```python
from build123d import *

# Parameters (mm, degrees)
SKETCH3_W           = 145
SKETCH3_H           = 90
SKETCH3_W_2         = 141.777777778
SKETCH3_H_2         = 88
BOSS_EXTRUDE1_DEPTH = 110
SKETCH4_W           = 145
SKETCH4_H           = 90
BOSS_EXTRUDE2_DEPTH = 1
SKETCH5_W           = 12
SKETCH5_H           = 12
BOSS_EXTRUDE3_DEPTH = 110
SKETCH6_R           = 2
CUT_EXTRUDE1_DEPTH  = 12
SKETCH7_R           = 10
CUT_EXTRUDE2_DEPTH  = 12


with BuildPart() as part:
    # Sketch3 → Boss-Extrude1 (new body)
    with BuildSketch(Plane(origin=(0, 0, 0), x_dir=(1, 0, 0), z_dir=(0, 1, 0))):
        Rectangle(SKETCH3_W, SKETCH3_H)
        Rectangle(SKETCH3_W_2, SKETCH3_H_2, mode=Mode.SUBTRACT)
    extrude(amount=BOSS_EXTRUDE1_DEPTH)

    # Sketch4 → Boss-Extrude2 (add)
    with BuildSketch(Plane.XZ):
        Rectangle(SKETCH4_W, SKETCH4_H)
    extrude(amount=BOSS_EXTRUDE2_DEPTH)

    # Sketch5 → Boss-Extrude3 (add)
    with BuildSketch(Plane(origin=(0, 0, 0), x_dir=(1, 0, 0), z_dir=(0, 1, 0))):
        with Locations((-64.888888889, 38)):
            Rectangle(SKETCH5_W, SKETCH5_H)
        with Locations((64.888888889, 38)):
            Rectangle(SKETCH5_W, SKETCH5_H)
        with Locations((64.888888889, -38)):
            Rectangle(SKETCH5_W, SKETCH5_H)
        with Locations((-64.888888889, -38)):
            Rectangle(SKETCH5_W, SKETCH5_H)
    extrude(amount=BOSS_EXTRUDE3_DEPTH)

    # Sketch6 → Cut-Extrude1 (cut)
    with BuildSketch(Plane(origin=(0, 110, 0), x_dir=(1, 0, 0), z_dir=(0, 1, 0))):
        with Locations((-67.5, 40)):
            Circle(SKETCH6_R)
        with Locations((-67.5, -40)):
            Circle(SKETCH6_R)
        with Locations((67.5, -40)):
            Circle(SKETCH6_R)
        with Locations((67.5, 40)):
            Circle(SKETCH6_R)
    extrude(amount=-CUT_EXTRUDE1_DEPTH, mode=Mode.SUBTRACT)

    # Sketch7 → Cut-Extrude2 (cut)
    with BuildSketch(Plane(origin=(0, 0, 0), x_dir=(1, 0, 0), z_dir=(0, 1, 0))):
        Circle(SKETCH7_R)
    extrude(amount=-CUT_EXTRUDE2_DEPTH, mode=Mode.SUBTRACT)


solid = part.part
```
Check sheet for the modelled part. Datum: model origin and axes. Units: mm. A direction names the side the tool comes from. Give positions to 0.01 mm unless a question says otherwise; leave off trailing zeros. Order: outer loops, then holes, each group sorted by start corner. A loop starts at its lowest first (then second) coordinate and runs counter-clockwise, first axis right, second up. Notation, with made-up numbers: M -38,10 L -24,10 A12 ccw -24,22 Z; hole C 15.25,39 d10. An arc over 180 degrees is marked long. Answer in a Markdown table with one row per item. Add a question column.
Q1. Access from +Z, -Z, +X, -X, +Y, -Y to the whole of each face (thin tool, end or side, straight path). Record for faces 4 (the cylindrical face through (-2.17, -0.49, 9.76)), 5 (the flat face through (65, 54, -32)).
Q2. Sectioned sample at A-A, the plane x = 0. Record the boundary of the cut face in (y, z), and give its area (3 significant figures).
Q3. Release check for a two-part mould opening along Z. For faces 1 (the flat face through (-58.889, 54, -38)), 2 (the flat face through (-1, -1, 11)), 3 (the flat face through (-1, 55, -45)) record: released by +Z, released by -Z, zero draft, split by the parting line, or undercut.
Q4. Sectioned sample at B-B, the plane z = 0. Record the boundary of the cut face in (x, y), and give its area (3 significant figures).
Q5. Sectioned sample at D-D, the plane z = -35. Record the boundary of the cut face in (x, y), and give its area (3 significant figures).
Q6. Thickness scan on L1, parallel to X at y = 102.5, z = 40; L2, parallel to Z at x = -67.5, y = 103.25; L3, parallel to X at y = 6.5, z = -24. Record the ranges inside material, lowest first.
Q7. Sectioned sample at C-C, the plane y = 34. Record the boundary of the cut face in (x, z), and give its area (3 significant figures).
Q8. Gauge pin test, flat ends, axial feed: pin 1 Ø23 at (x, z) = (0, 0) entering from +Y; pin 2 Ø6 at (x, z) = (6.5, 1) entering from +Y. Record the tip position at first contact, or that the pin passes through.
Verdict:
| question | item | result |
|---|---|---|
| 1 | face 4 | +Y, -Y |
| 1 | face 5 | +Y |
| 2 | outline | M -1,-45 L 110,-45 L 110,-44 L 0,-44 L 0,-10 L -1,-10 Z; M -1,10 L 0,10 L 0,44 L 110,44 L 110,45 L -1,45 Z |
| 2 | area | 290 mm² |
| 3 | face 1 | undercut |
| 3 | face 2 | zero draft |
| 3 | face 3 | released by -Z |
| 4 | outline | M -72.5,-1 L -10,-1 L -10,0 L -70.89,0 L -70.89,110 L -72.5,110 Z; M 10,-1 L 72.5,-1 L 72.5,110 L 70.89,110 L 70.89,0 L 10,0 Z |
| 4 | area | 479 mm² |
| 5 | outline | M -72.5,-1 L 72.5,-1 L 72.5,110 L 58.89,110 L 58.89,0 L -58.89,0 L -58.89,110 L -72.5,110 Z |
| 5 | area | 3,140 mm² |
| 6 | L1 | -72.5 to -69.5, -65.5 to -58.89, 58.89 to 65.5, 69.5 to 72.5 |
| 6 | L2 | -45 to -42, -38 to -32, 32 to 38, 42 to 45 |
| 6 | L3 | -72.5 to -70.89, 70.89 to 72.5 |
| 7 | outline | M -72.5,-45 L 72.5,-45 L 72.5,45 L -72.5,45 Z; hole M -70.89,-32 L -58.89,-32 L -58.89,-44 L 58.89,-44 L 58.89,-32 L 70.89,-32 L 70.89,32 L 58.89,32 L 58.89,44 L -58.89,44 L -58.89,32 L -70.89,32 Z |
| 7 | area | 1,150 mm² |
| 8 | pin 1 | y = 0 |
| 8 | pin 2 | through |
